Solid Edge part; units mm, degrees
sketch "Sketch1" plane through (0, 0, 0) normal (0, 0, 1) x (1, 0, 0)
  circle A0 centre (0, 0) radius 2.5
extrude "Protrusion1" add sketch "Sketch1" against normal blind 1.5
sketch "Sketch2" plane through (0, 0, -1.5) normal (0, 0, -1) x (1, 0, 0)
  circle A0 centre (0, 0) radius 4
extrude "ExtrudedProtrusion_2" add sketch "Sketch2" along normal blind 4
fillet "Round_1" radius 2 1 edges at (-4, 0, -5.5)
properties material "ABS Plastic, medium impact"
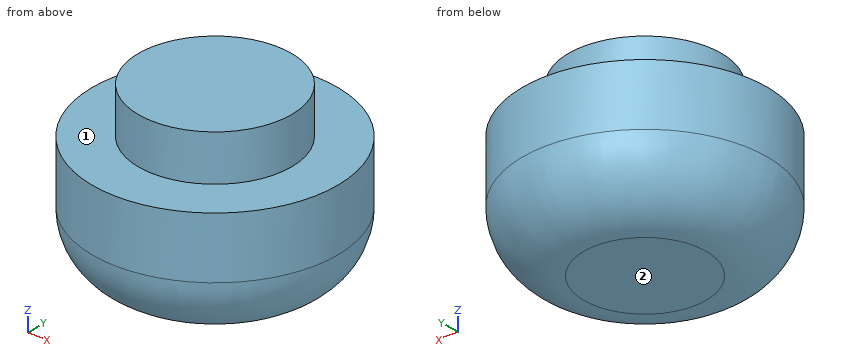
Could you check a few things on this model? Use its own coordinates, in mm. Face numbers are marked on the shaded views. A direction names the side the tool comes from. Round coordinates to 2 decimals unless told otherwise and drop trailing zeros. Loops run counter-clockwise (first coordinate to the right, second up) from the corner with the lowest first, then second, coordinate; pieces in that order, holes last. Notation, with made-up numbers: M -6,45.5 L 53,45.5 A20 cw 53,58.5 Z; hole C 6,15.5 d11. An arc over 180 degrees is marked long. Write item = value, one per line.
1. Will these pins go through, and if not, where does the flat tip stop? P1, Ø2, axis at x = -2.5, y = 3, coming from the +Z side; P2, Ø1, axis at y = 2.5, z = -1.5, coming from the +X side.
Results below:
P1 = -1.5
P2 = 3.46
2. I want a section at B-B, the plane z = -1.35. Write out the boundary of the cut face in (x, y).
Results below:
outline = C 0,0 d5
3. I need wall thicknesses on probe 1 along Y at (x, z) = (0, -3.55); probe 2 along X at (y, z) = (-1.5, -1.25); probe 3 along Y at (x, z) = (-1.5, -4). Which ranges of each line are inside material? Lowest first, please.
Results below:
probe_1 = -4 to 4
probe_2 = -2 to 2
probe_3 = -3.64 to 3.64
4. Which directions (+Z, -Z, +X, -X, +Y, -Y) give clear straight access to the entire face, cutting with the end or side of a thin tool? Please do the marked faces 1 and 2.
Results below:
face_1 = +Z
face_2 = -Z, +X, -X, +Y, -Y
5. I want a section at A-A, the plane z = -2.05. Write out the boundary of the cut face in (x, y), and give its area (3 significant figures).
Results below:
outline = C 0,0 d8
area = 50.3 mm²
